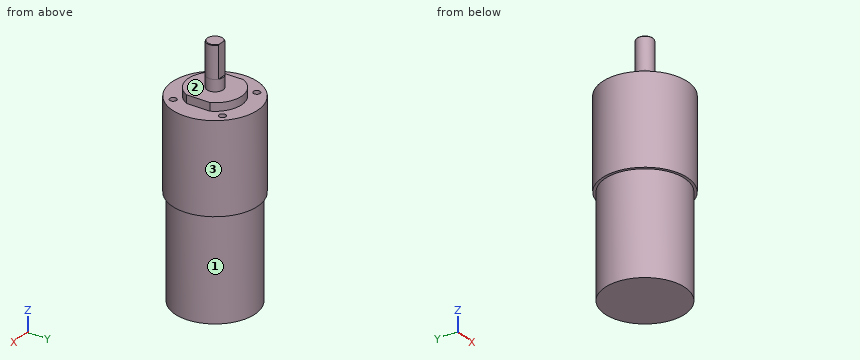
```python
from build123d import *

# Parameters (mm, degrees)
F0_R      = 15
F1_DEPTH  = 37.8
F2_R      = 16
F3_DEPTH  = 33.4
F5_DEPTH  = 3
F6_R      = 3
F7_DEPTH  = 4.3
F9_DEPTH  = 12
F10_SIZE  = 0.2
F11_R     = 1.25
F12_DEPTH = 5.5


with BuildPart() as f1:
    # F0 (on Top) → F1 (new body)
    with BuildSketch(Plane.XY):
        Circle(F0_R)
    extrude(amount=F1_DEPTH)

    # F2 (on face) → F3 (join)
    with BuildSketch(Plane.XY.offset(37.8)):
        Circle(F2_R)
    extrude(amount=F3_DEPTH)

    # F4 (on face) → F5 (join)
    with BuildSketch(Plane.XY.offset(71.2)):
        with BuildLine():
            Line((-9, 4.3588989435), (-9, -4.3588989435))
            ThreePointArc((-9, -4.3588989435), (0, -10), (9, -4.3588989435))
            Line((9, -4.3588989435), (9, 4.3588989435))
            ThreePointArc((9, 4.3588989435), (0, 10), (-9, 4.3588989435))
        make_face()
    extrude(amount=F5_DEPTH)

    # F6 (on face) → F7 (join)
    with BuildSketch(Plane.XY.offset(74.2)):
        Circle(F6_R)
    extrude(amount=F7_DEPTH)

    # F8 (on face) → F9 (join)
    with BuildSketch(Plane.XY.offset(78.5)):
        with BuildLine():
            Line((1.6583123952, 2.5), (-1.6583123952, 2.5))
            ThreePointArc((-1.6583123952, 2.5), (0, -3), (1.6583123952, 2.5))
        make_face()
    extrude(amount=F9_DEPTH)

    # F10
    f10_edges = [f1.edges().sort_by_distance(p)[0] for p in [
        (0, -3, 90.5),
    ]]
    chamfer(f10_edges, length=F10_SIZE)

    # F11 (on face) → F12 (cut)
    with BuildSketch(Plane.XY.offset(71.2)):
        with Locations((9.1923881554, -9.1923881554)):
            Circle(F11_R)
        with Locations((-9.1923881554, -9.1923881554)):
            Circle(F11_R)
        with Locations((9.1923881554, 9.1923881554)):
            Circle(F11_R)
        with Locations((-9.1923881554, 9.1923881554)):
            Circle(F11_R)
    extrude(amount=-F12_DEPTH, mode=Mode.SUBTRACT)


solid = f1.part
```
The model under review builds one solid part; all positions refer to its coordinate system, in mm. Face numbers are marked on the shaded views. A direction names the side the tool comes from. Coordinates: 2 decimals unless noted, no trailing zeros. Loops run counter-clockwise (first coordinate to the right, second up) from the corner with the lowest first, then second, coordinate; pieces in that order, holes last. Notation, with made-up numbers: (-10, 66) -> (-4, 66) arc R23 cw to (-4, 78) -> close; hole circle Ø9 at (-3.75, -10). An arc over 180 degrees is marked (long way). Answer as CSV lines item,"result".
Item 1: Take a section at C-C, the plane z = 68.5. State the section outline as (x, y) points, and give its area (3 significant figures).
Results below:
outline,"circle Ø32 at (0, 0); hole circle Ø2.5 at (-9.19, -9.19); hole circle Ø2.5 at (-9.19, 9.19); hole circle Ø2.5 at (9.19, -9.19); hole circle Ø2.5 at (9.19, 9.19)"
area,"785 mm2"
Item 2: Insertion check: pin 1 (2.5 mm diameter, centred on x = -1, z = 84, fed in from +Y); pin 2 (1.5 mm diameter, centred on y = 1, z = 72.5, fed in from -X); pin 3 (0.8 mm diameter, centred on x = -9, y = -9, fed in from +Z); pin 4 (10 mm diameter, centred on y = -4, z = 71.5, fed in from +X). Each pin has a flat end and moves straight along its axis. Give the tip position at first contact, or say it passes through.
Results below:
pin 1,"stops at y = 2.5"
pin 2,"stops at x = -9"
pin 3,"stops at z = 65.7"
pin 4,"stops at x = 16"
Item 3: Machinability: for the marked faces 1, 2 and 3, which of the approach directions +Z, -Z, +X, -X, +Y, -Y give a long, thin tool a straight path to every point of the face, cutting with its end or side? Answer none if there is none.
Results below:
face 1,"-Z"
face 2,"+Z"
face 3,"+Z, -Z"
Item 4: Take a section at A-A, the plane y = 0. State the section outline as (x, z) points, and give its area (3 significant figures).
Results below:
outline,"(-16, 37.8) -> (-15, 37.8) -> (-15, 0) -> (15, 0) -> (15, 37.8) -> (16, 37.8) -> (16, 71.2) -> (9, 71.2) -> (9, 74.2) -> (3, 74.2) -> (3, 90.3) -> (2.8, 90.5) -> (-2.8, 90.5) -> (-3, 90.3) -> (-3, 74.2) -> (-9, 74.2) -> (-9, 71.2) -> (-16, 71.2) -> close"
area,"2,350 mm2"
Item 5: Take a section at B-B, the plane x = 13. State the section outline as (y, z) points, and give its area (3 significant figures).
Results below:
outline,"(-9.33, 37.8) -> (-7.48, 37.8) -> (-7.48, 0) -> (7.48, 0) -> (7.48, 37.8) -> (9.33, 37.8) -> (9.33, 71.2) -> (-9.33, 71.2) -> close"
area,"1,190 mm2"
Item 6: For L1, parallel to Y at x = -9, z = 70.5; L2, parallel to Z at x = 3, y = 12; L3, parallel to Z at x = -0.5, y = -3, list the stretches that pass through material, from the lowest coordinate up.
Results below:
L1,"y = -13.23 to -10.43, -7.96 to 7.96, 10.43 to 13.23"
L2,"z = 0 to 71.2"
L3,"z = 0 to 74.2"
Item 7: Take a section at D-D, the plane z = 42. State the section outline as (x, y) points, and give its area (3 significant figures).
Results below:
outline,"circle Ø32 at (0, 0)"
area,"804 mm2"
